```python
from build123d import *

# Parameters (mm, degrees)
SKETCH1_R           = 1.778
SKETCH1_R_2         = 3.175
BOSS_EXTRUDE1_DEPTH = 4.7625


with BuildPart() as part:
    # Sketch1 → Boss-Extrude1 (new body)
    with BuildSketch(Plane(origin=(0, 0, 0), x_dir=(1, 0, 0), z_dir=(0, 1, 0))):
        with BuildLine():
            Line((-38.770225031, 16.757963615), (-43.625448569, 14.598747375))
            ThreePointArc((-43.625448569, 14.598747375), (-45.155674622, 14.559326862), (-46.265582353, 15.613485569))
            Line((-46.265582353, 15.613485569), (-47.282683039, 17.900542834))
            ThreePointArc((-47.282683039, 17.900542834), (-47.541465806, 19.100109045), (-47.298283286, 20.302934833))
            ThreePointArc((-47.298283286, 20.302934833), (-45.865213893, 23.360627542), (-44.234733225, 26.317772344))
            ThreePointArc((-44.234733225, 26.317772344), (-39.855484626, 29.811728531), (-34.259632886, 29.543416329))
            Line((-34.259632886, 29.543416329), (5.363638877, 12.388760148))
            ThreePointArc((5.363638877, 12.388760148), (7.44200849, -11.263503435), (-13.499793526, -0.074664302))
            Line((-13.499793526, -0.074664302), (-36.286855081, 16.495885282))
            ThreePointArc((-36.286855081, 16.495885282), (-37.403602541, 17.810792136), (-38.770225031, 16.757963615))
        make_face()
        with Locations((-20.862458922, 15.093717491)):
            Circle(SKETCH1_R, mode=Mode.SUBTRACT)
        Circle(SKETCH1_R_2, mode=Mode.SUBTRACT)
        with Locations((-37.413253893, 22.259284205)):
            Circle(SKETCH1_R, mode=Mode.SUBTRACT)
    extrude(amount=BOSS_EXTRUDE1_DEPTH)


solid = part.part
```
Source: CAD feature listing. Evaluate the final solid. Frame: model axes, mm. A direction names the side the tool comes from. Give positions to 0.01 mm unless a question says otherwise; leave off trailing zeros. Order: outer loops, then holes, each group sorted by start corner. A loop starts at its lowest first (then second) coordinate and runs counter-clockwise, first axis right, second up.
(1) Material intervals for line 1 along X through (y, z) = (1.95, -16); line 2 along X through (y, z) = (1.5, 0) (3 decimals); line 3 along Z through (x, y) = (0, 3.8) (3 decimals), sorted ascending.
(2) Section query C-C (y = 1.1). State how many separate pieces and enclosed holes the cut face has, plus the area to 3 significant figures.
(3) Access query for faces 4 (the face through (-45.887, 2.348, -23.318)), 5 (the face through (-41.164, 2.348, -15.693)). Directions: +Z, -Z, +X, -X, +Y, -Y. A direction counts if a zero-diameter tool reaches every point of the face in a straight line with its end or side. Return the directions, or none.
(4) Section query B-B (x = 0). Return the cut outline in (y, z) (1 decimal), plus the area to 3 significant figures.
(5) Pull-direction query (Z, two-part tool) for faces 1 (the face through (-47.54, 2.35, -19.08)), 2 (the face through (-39.932, 2.348, -29.787)), 3 (the face through (-20.042, 2.348, -13.516)); classes: +Z half, -Z half, draft (parallel to the pull), parting line (faces both ways), or undercut.
(6) Section query A-A (z = 2.5). Return the cut outline in (x, y), plus the area to 3 significant figures.
(7) Contact query for flat-ended pins moving along their axis: P1, Ø2, axis at y = 4, z = -17, coming from the -X side; P2, Ø2, axis at x = -20.86, z = -15.09, coming from the +Y side; P3, Ø1, axis at y = 1.5, z = 6.5, coming from the -X side; P4, Ø1, axis at x = 5.5, y = 2.5, coming from the +Z side. Output: stop coordinate, or through.
(8) Section query D-D (x = -40.5). Return the cut outline in (y, z), plus the area to 3 significant figures.
Outcome:
1. line 1: x = -46.44 to -40.47, -35.6 to -22.39, -19.33 to -2.98
1. line 2: x = -13.602 to -3.175, 3.175 to 13.5
1. line 3: z = -14.711 to -3.175, 3.175 to 13.5
2. separate pieces: 1
2. enclosed holes: 3
2. area: 1,140 mm2
3. face 4: -Z, -X, +Y, -Y
3. face 5: +Z, +Y, -Y
4. outline: (0, -14.7) - (4.8, -14.7) - (4.8, -3.2) - (0, -3.2) - close; (0, 3.2) - (4.8, 3.2) - (4.8, 13.5) - (0, 13.5) - close
4. area: 104 mm2
5. face 1: parting line
5. face 2: -Z half
5. face 3: undercut
6. outline: (-13.27, 0) - (-1.96, 0) - (-1.96, 4.76) - (-13.27, 4.76) - close; (1.96, 0) - (13.27, 0) - (13.27, 4.76) - (1.96, 4.76) - close
6. area: 108 mm2
7. P1: stops at x = -47.32
7. P2: passes through
7. P3: stops at x = -12.09
7. P4: stops at z = 12.54
8. outline: (0, -29.57) - (4.76, -29.57) - (4.76, -15.99) - (0, -15.99) - close
8. area: 64.7 mm2
